Autodesk Inventor part; units mm, degrees
ref_plane "YZ Plane" through (0, 0, 0) normal (1, 0, 0) x (0, 1, 0)
ref_plane "XZ Plane" through (0, 0, 0) normal (0, 1, 0) x (-1, 0, 0)
ref_plane "XY Plane" through (0, 0, 0) normal (0, 0, 1) x (1, 0, 0)
sketch "Esquisse1" plane through (0, 0, 0) normal (0, 0, 1) x (1, 0, 0)
  line L0 (-40, 30) -> (40, 30)
  line L1 (40, 30) -> (40, -17)
  line L2 (40, -17) -> (-40, -17)
  line L3 (-40, -17) -> (-40, 30)
  point P0 (0, 0)
  dimension "d0" = 47
  dimension "d1" = 80
  dimension "d2" = 40
  dimension "d3" = 30
extrude "Extrusion1" add sketch "Esquisse1" along normal blind 40
sketch "Esquisse2" plane through (0, 0, 40) normal (0, 0, 1) x (1, 0, 0)
  circle A0 centre (0, 5) radius 18
  line L0 (40, -17) -> (40, 30)
  line L1 (-40, 30) -> (40, 30)
  point P0 (0, 0)
  dimension "d6" = 36
  dimension "d7" = 40
  dimension "d8" = 25
extrude "Extrusion2" cut sketch "Esquisse2" against normal blind 40
sketch "Esquisse3" plane through (0, 0, 40) normal (0, 0, 1) x (1, 0, 0)
  circle A0 centre (0, 5) radius 18
  line L0 (40, -17) -> (-40, -17)
  line L1 (-25, -17) -> (25, -17)
  line L2 (25, -17) -> (25, 9)
  line L3 (-25, 9) -> (-25, -17)
  line L4 (-25, 9) -> (-17, 17)
  line L5 (17, 17) -> (25, 9)
  line L6 (17, 17) -> (13.4164, 17)
  line L7 (-13.4164, 17) -> (-17, 17)
  point P0 (0, 0)
  point P1 (25, 17)
  point P2 (-25, 17)
extrude "Extrusion3" cut sketch "Esquisse3" against normal blind 40
sketch "Esquisse4" plane through (-40, -17, 0) normal (0, -1, 0) x (1, 0, 0)
  line L0 (8, 10) -> (72, 10)
  line L1 (72, 10) -> (72, 30)
  line L2 (72, 30) -> (8, 30)
  line L3 (8, 30) -> (8, 10)
  line L4 (0, 40) -> (80, 40)
  line L5 (80, 0) -> (0, 0)
  point P0 (40, 0)
  point P1 (15, 40)
  point P2 (65, 0)
  dimension "d23" = 64
  dimension "d24" = 32
  dimension "d25" = 10
  dimension "d26" = 10
hole "Perçage1" at (-32, -17, 30) at (32, -17, 30) at (32, -17, 10) at (-32, -17, 10) direction (0, 1, 0) diameter 4 depth 100 tip angle 118
sketch "Esquisse5" plane through (-40, 30, 0) normal (0, 1, 0) x (1, 0, 0)
  circle A0 centre (72, -30) radius 2
  line L0 (8, -10) -> (72, -10)
  line L1 (72, -10) -> (72, -30)
  line L2 (72, -30) -> (8, -30)
  line L3 (8, -30) -> (8, -10)
  circle A1 centre (8, -10) radius 2
  line L4 (8, -20) -> (72, -20)
  point P0 (40, 0)
hole "Perçage2" at (-32, 30, 10) at (-32, 30, 20) at (-32, 30, 30) at (32, 30, 30) at (32, 30, 20) at (32, 30, 10) direction (0, -1, 0) diameter 4 depth 100 tip angle 118 counterbore diameter 6 counterbore depth 43
chamfer "Chanfrein2" distance 18 distance2 18 1 edges at (40, 30, 20)
chamfer "Chanfrein3" distance 18 distance2 18 1 edges at (-40, 30, 20)
properties part number "Soutient_Mot"
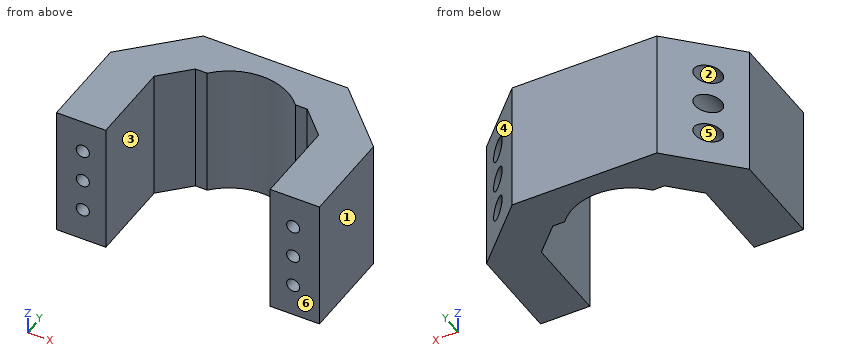
Part model, mm, in its own coordinate system. Face numbers are marked on the shaded views. A direction names the side the tool comes from. Give positions to 0.01 mm unless a question says otherwise; leave off trailing zeros. Loops run counter-clockwise (first coordinate to the right, second up) from the corner with the lowest first, then second, coordinate; pieces in that order, holes last.
(1) Pull direction X, two halves, no side cores. Call the marked faces 4, 5 and 6: pulls with the +X half, pulls with the -X half, needs draft (parallel to the pull), parting line crosses it, or undercut.
Return value:
face 4: pulls with the +X half
face 5: undercut
face 6: needs draft
(2) Pin check, flat tips, straight feed: pin 1 (1.8 mm diameter, centred on x = 33, z = 28.5, fed in from +Y); pin 2 (6.5 mm diameter, centred on x = -31, z = 11, fed in from +Y); pin 3 (6.5 mm diameter, centred on x = 32, z = 30, fed in from +Y). Stop position of each tip, or through.
Return value:
pin 1: stops at y = -13
pin 2: stops at y = 24.25
pin 3: stops at y = 23.25
(3) 3-axis set-ups, long thin cutter, end or side, ignore diameter. For the marked faces 1, 2 and 3: which of +Z, -Z, +X, -X, +Y, -Y reach the whole face in a straight line?
Return value:
face 1: +Z, -Z, +X, +Y, -Y
face 2: +Y
face 3: +Z, -Z, -Y
(4) Band-saw the part on B-B (z = 30). Count the separate pieces of the cut face and the enclosed holes in it, and give its area (3 significant figures).
Return value:
separate pieces: 3
enclosed holes: 0
area: 1,260 mm2
(5) Band-saw the part on A-A (y = 13.5). Write the cut outline in (x, z), and give its area (3 significant figures).
Return value:
outline: (-38.5, 0) - (-20.5, 0) - (-20.5, 40) - (-38.5, 40) - close; (20.5, 0) - (38.5, 0) - (38.5, 40) - (20.5, 40) - close; hole circle Ø6 at (-32, 10); hole circle Ø6 at (-32, 20); hole circle Ø6 at (-32, 30); hole circle Ø6 at (32, 10); hole circle Ø6 at (32, 20); hole circle Ø6 at (32, 30)
area: 1,270 mm2
(6) Band-saw the part on C-C (x = -32). Write the cut outline in (y, z), and give its area (3 significant figures).
Return value:
outline: (-17, 0) - (20, 0) - (20, 7) - (-13, 7) - (-13, 8) - (-17, 8) - close; (-17, 12) - (-13, 12) - (-13, 13) - (20, 13) - (20, 17) - (-13, 17) - (-13, 18) - (-17, 18) - close; (-17, 22) - (-13, 22) - (-13, 23) - (20, 23) - (20, 27) - (-13, 27) - (-13, 28) - (-17, 28) - close; (-17, 32) - (-13, 32) - (-13, 33) - (20, 33) - (20, 40) - (-17, 40) - close
area: 838 mm2
(7) Band-saw the part on D-D (y = -3.5). Write the cut outline in (x, z), and give its area (3 significant figures).
Return value:
outline: (-40, 0) - (-25, 0) - (-25, 40) - (-40, 40) - close; (25, 0) - (40, 0) - (40, 40) - (25, 40) - close; hole circle Ø6 at (-32, 10); hole circle Ø6 at (-32, 20); hole circle Ø6 at (-32, 30); hole circle Ø6 at (32, 10); hole circle Ø6 at (32, 20); hole circle Ø6 at (32, 30)
area: 1,030 mm2
(8) Drill centre lines: line 1 along Z through (x, y) = (32, -14); line 2 along X through (y, z) = (-15, 10); line 3 along X through (y, z) = (4, 10). Where is each one in solid material? Low to high.
Return value:
line 1: z = 0 to 8, 12 to 18, 22 to 28, 32 to 40
line 2: x = -40 to -34, -30 to -25, 25 to 30, 34 to 40
line 3: x = -40 to -35, -29 to -25, 25 to 29, 35 to 40
